Check sheet for the modelled part. Datum: model origin and axes. Units: mm. Round coordinates to 2 decimals unless told otherwise and drop trailing zeros. Write each loop counter-clockwise with the first axis right and the second up, starting at its lowest first coordinate (ties: lowest second). Pieces come first, ordered by that corner, then holes. Notation, with made-up numbers: M 7.5,-30 L 30.5,-30 A7 ccw 30.5,-23 Z; hole C 0.5,-37.75 d11. An arc over 180 degrees is marked long. One line per item, written item: value.
Autodesk Inventor part; units mm, degrees
ref_plane "YZ Plane" through (0, 0, 0) normal (1, 0, 0) x (0, 1, 0)
ref_plane "XZ Plane" through (0, 0, 0) normal (0, 1, 0) x (-1, 0, 0)
ref_plane "XY Plane" through (0, 0, 0) normal (0, 0, 1) x (1, 0, 0)
sketch "스케치1" plane through (0, 0, 0) normal (0, 1, 0) x (-1, 0, 0)
  line L0 (0, 0) -> (-40, 0)
  line L1 (-40, 0) -> (-40, -270)
  line L2 (-40, -270) -> (0, -270)
  line L3 (0, -270) -> (0, 0)
  dimension "d0" = 40
  dimension "d1" = 270
extrude "돌출1" add sketch "스케치1" along normal blind 2
sketch "스케치2" plane through (0, 2, 0) normal (0, 1, 0) x (1, 0, 0)
  line L0 (0, 0) -> (40, 0)
  line L1 (40, 0) -> (40, 270)
  line L2 (40, 270) -> (0, 270)
  line L3 (0, 270) -> (0, 0)
  line L4 (0, 270) -> (0, 0)
  line L5 (40, 229) -> (0, 229)
  line L6 (0, 229) -> (0, 220.8)
  line L7 (0, 220.8) -> (40, 220.8)
  line L8 (40, 220.8) -> (40, 229)
  line L9 (40, 0) -> (40, 270)
  line L10 (40, 49.2) -> (0, 49.2)
  line L11 (0, 49.2) -> (0, 41)
  line L12 (0, 41) -> (40, 41)
  line L13 (40, 41) -> (40, 49.2)
  dimension "d4" = 8.2
  dimension "d5" = 8.2
  dimension "d6" = 41
  dimension "d7" = 41
extrude "돌출2" cut sketch "스케치2" against normal blind 1 contours L3 L10 L1 L12 | L3 L5 L1 L7
sketch "스케치3" plane through (0, 0, 0) normal (0, -1, 0) x (1, 0, 0)
  line L0 (0, 0) -> (40, 0)
  line L1 (0, -270) -> (0, 0)
  line L2 (40, -270) -> (0, -270)
  line L3 (40, 0) -> (40, -270)
  line L4 (37, -260) -> (37, -190)
  line L5 (37, -190) -> (23, -190)
  line L6 (23, -190) -> (23, -260)
  line L7 (23, -80) -> (37, -80)
  line L8 (37, -80) -> (37, -10)
  line L9 (37, -10) -> (23, -10)
  line L10 (23, -10) -> (23, -80)
  line L11 (23, -260) -> (37, -260)
  dimension "d15" = 14
  dimension "d17" = 3
  dimension "d20" = 14
  dimension "d21" = 70
  dimension "d22" = 3
  dimension "d23" = 10
  dimension "d25" = 10
  dimension "d26" = 70
extrude "돌출4" cut sketch "스케치3" against normal blind 2 contours L11 L6 L5 L4 | L10 L9 L8 L7
sketch "스케치4" plane through (0, 0, 0) normal (0, -1, 0) x (1, 0, 0)
  line L0 (23, -190) -> (37, -190)
  line L1 (37, -190) -> (37, -260)
  line L2 (37, -260) -> (23, -260)
  line L3 (23, -260) -> (23, -190)
  line L4 (37, -10) -> (37, -80)
  line L5 (37, -80) -> (23, -80)
  line L6 (23, -80) -> (23, -10)
  line L7 (23, -10) -> (37, -10)
  line L8 (0, 0) -> (40, 0)
  line L9 (0, -270) -> (0, 0)
  line L10 (40, -270) -> (0, -270)
  line L11 (40, 0) -> (40, -270)
  line L12 (23, -175) -> (37, -175)
  line L13 (37, -95) -> (23, -95)
  line L14 (23, -95) -> (23, -175)
  line L15 (37, -95) -> (37, -175)
  dimension "d36" = 95
  dimension "d39" = 14
  dimension "d40" = 3
  dimension "d41" = 80
extrude "돌출6" cut sketch "스케치4" against normal blind 2 contours L14 L13 L15 L12
sketch "스케치5" plane through (0, 2, 0) normal (0, 1, 0) x (1, 0, 0)
  line L0 (40, 229) -> (40, 270)
  line L1 (0, 270) -> (0, 229)
  line L2 (40, 269) -> (0, 269)
  line L3 (0, 269) -> (0, 260.8)
  line L4 (0, 260.8) -> (40, 260.8)
  line L5 (40, 260.8) -> (40, 269)
  line L6 (40, 0) -> (40, 41)
  line L7 (0, 41) -> (0, 0)
  line L8 (40, 9.2) -> (0, 9.2)
  line L9 (0, 9.2) -> (0, 1)
  line L10 (0, 1) -> (40, 1)
  line L11 (40, 1) -> (40, 9.2)
  line L12 (0, 0) -> (40, 0)
  line L13 (40, 270) -> (0, 270)
  dimension "d44" = 8.2
  dimension "d45" = 8.2
  dimension "d46" = 1
  dimension "d47" = 1
extrude "돌출7" cut sketch "스케치5" against normal blind 1 contours L4 L1 L2 L0 | L10 L7 L8 L6
sketch "스케치6" plane through (0, 0, 0) normal (0, -1, 0) x (1, 0, 0)
  line L0 (0, -9.2) -> (40, -9.2)
  line L1 (40, -9.2) -> (40, -41)
  line L2 (40, -41) -> (37, -41)
  line L3 (37, -41) -> (37, -10)
  line L4 (37, -10) -> (23, -10)
  line L5 (23, -10) -> (23, -41)
  line L6 (23, -41) -> (0, -41)
  line L7 (0, -41) -> (0, -9.2)
  line L8 (37, -95) -> (23, -95)
  line L9 (23, -190) -> (23, -220.8)
  line L10 (23, -220.8) -> (0, -220.8)
  line L11 (0, -220.8) -> (0, -49.2)
  line L12 (0, -49.2) -> (23, -49.2)
  line L13 (23, -49.2) -> (23, -80)
  line L14 (23, -80) -> (37, -80)
  line L15 (37, -80) -> (37, -49.2)
  line L16 (37, -49.2) -> (40, -49.2)
  line L17 (40, -49.2) -> (40, -220.8)
  line L18 (40, -220.8) -> (37, -220.8)
  line L19 (37, -220.8) -> (37, -190)
  line L20 (40, -260.8) -> (0, -260.8)
  line L21 (0, -260.8) -> (0, -229)
  line L22 (0, -229) -> (23, -229)
  line L23 (23, -229) -> (23, -260)
  line L24 (23, -260) -> (37, -260)
  line L25 (37, -260) -> (37, -229)
  line L26 (37, -229) -> (40, -229)
  line L27 (40, -229) -> (40, -260.8)
  line L28 (0, -269) -> (40, -269)
  line L29 (40, -269) -> (40, -270)
  line L30 (40, -270) -> (0, -270)
  line L31 (0, -270) -> (0, -269)
  line L32 (40, -1) -> (0, -1)
  line L33 (0, -1) -> (0, 0)
  line L34 (0, 0) -> (40, 0)
  line L35 (40, 0) -> (40, -1)
  circle A0 centre (6, -5.1) radius 1.5
  circle A1 centre (16, -5.1) radius 1.5
  circle A2 centre (6, -45.1) radius 1.5
  circle A3 centre (16, -45.1) radius 1.5
  circle A4 centre (6, -224.9) radius 1.5
  circle A5 centre (16, -224.9) radius 1.5
  circle A6 centre (6, -264.9) radius 1.5
  circle A7 centre (16, -264.9) radius 1.5
  line L36 (0, -270) -> (0, 0)
  line L37 (37, -175) -> (37, -95)
  line L38 (23, -95) -> (23, -175)
  line L39 (23, -175) -> (37, -175)
  line L40 (37, -190) -> (23, -190)
  dimension "d50" = 3
  dimension "d51" = 3
  dimension "d52" = 3
  dimension "d53" = 3
  dimension "d54" = 3
  dimension "d55" = 3
  dimension "d56" = 3
  dimension "d57" = 3
  dimension "d58" = 4.1
  dimension "d59" = 6
  dimension "d60" = 4.1
  dimension "d61" = 10
  dimension "d62" = 4.1
  dimension "d63" = 4.1
  dimension "d64" = 6
  dimension "d65" = 10
  dimension "d66" = 4.1
  dimension "d67" = 4.1
  dimension "d68" = 6
  dimension "d69" = 10
  dimension "d70" = 4.1
  dimension "d71" = 4.1
  dimension "d72" = 6
  dimension "d73" = 10
extrude "돌출8" cut sketch "스케치6" against normal blind 3 contours A0 | A1 | A2 | A3 | A4 | A5 | A6 | A7
sketch "스케치8" plane through (0, 2, 0) normal (0, 1, 0) x (1, 0, 0)
  line L0 (39, 40) -> (38, 40)
  line L1 (22, 40) -> (0, 40)
  line L2 (39, 230) -> (38, 230)
  line L3 (22, 230) -> (0, 230)
  line L4 (0, 40) -> (40, 40)
  line L5 (40, 40) -> (40, 0)
  line L6 (40, 0) -> (0, 0)
  line L7 (0, 0) -> (0, 40)
  line L8 (40, 270) -> (0, 270)
  line L9 (0, 230) -> (40, 230)
  line L10 (40, 230) -> (40, 270)
  line L11 (40, 270) -> (0, 270)
  line L12 (0, 270) -> (0, 230)
extrude "돌출10" cut sketch "스케치8" against normal blind 2
properties part number "앞뒷판_위_수정" material "알루미늄 6061"
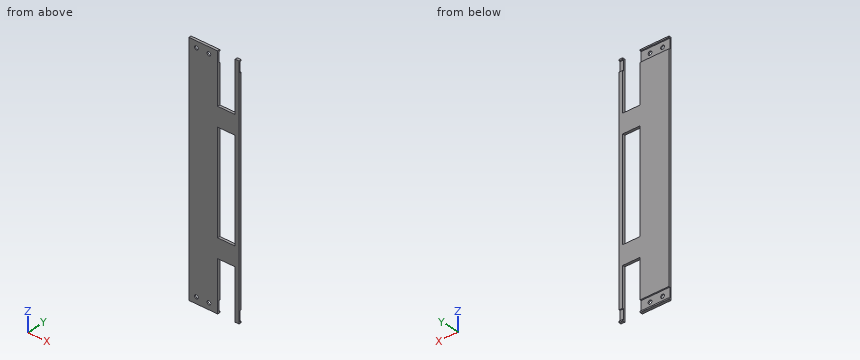
Q1. Sectioned sample at A-A on y = 1.6. State how many separate pieces and enclosed holes the cut face has, and give its area (3 significant figures).
Completed:
separate pieces: 5
enclosed holes: 1
area: 4,930 mm^2
Q2. Depth check by flat-ended pin: P1, Ø2.5, axis at x = 16, z = -224.9, coming from the +Y side; P2, Ø0.6, axis at x = 33, y = 1.5, coming from the -Z side; P3, Ø0.6, axis at x = 30, y = 0.5, coming from the +Z side; P4, Ø2.5, axis at x = 38, z = -43.5, coming from the +Y side. Enter the tip coordinate at first touch or a pass-through.
Completed:
P1: through
P2: z = -190
P3: z = -80
P4: y = 1
Q3. Sectioned sample at B-B on x = 31. Enter the section's corners in (y, z), and give its area (3 significant figures).
Completed:
outline: M 0,-190 L 2,-190 L 2,-175 L 0,-175 Z; M 0,-95 L 2,-95 L 2,-80 L 0,-80 Z
area: 60.0 mm^2
Q4. Scan lines: line 1 (X direction, y = 0.85, z = -224.9); line 2 (Z direction, x = 6, y = 0.3); line 3 (X direction, y = 0.35, z = -163). Record each from-to range of solid material in increasing order. Write a range as [from, to].
Completed:
line 1: [0, 4.5], [7.5, 14.5], [17.5, 23], [37, 40]
line 2: [-230, -226.4], [-223.4, -46.6], [-43.6, -40]
line 3: [0, 23], [37, 40]
